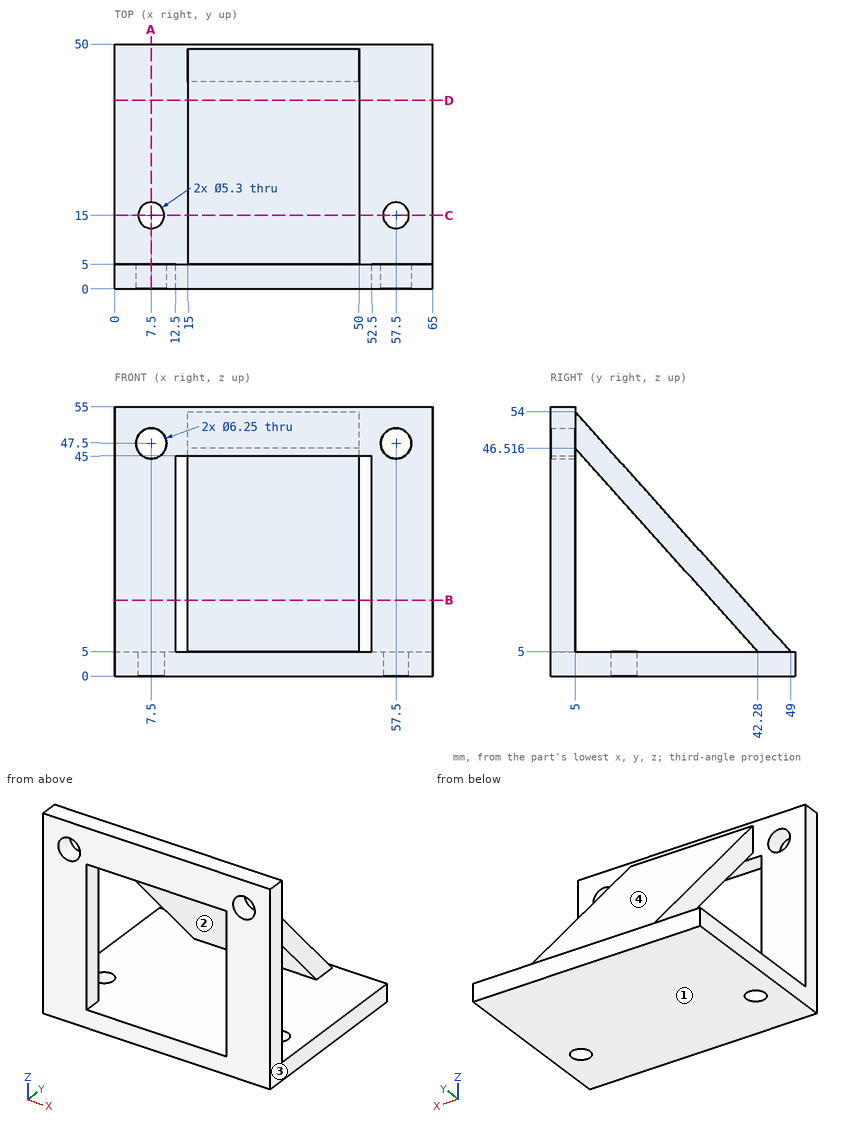
Answer from the drawing. Dimensions are ordinates in mm from the lowest x, y and z of the part. Give positions to 0.01 mm unless a question says otherwise; leave off trailing zeros. Write each loop counter-clockwise with the first axis right and the second up, starting at its lowest first coordinate (ties: lowest second). Pieces come first, ordered by that corner, then holes. Notation, with made-up numbers: (67.5, 52.5) - (110.5, 52.5) arc R22 cw to (110.5, 83.5) - close; hole circle Ø7 at (28, 28.25). An arc over 180 degrees is marked (long way). One line per item, written item: value. Start each with the question number.
1. Given pin 1 (12 mm diameter, centred on x = 40.5, y = 41.5, fed in from +Z) (1 decimal); pin 2 (1 mm diameter, centred on x = 55, z = 33, fed in from +Y); pin 3 (6 mm diameter, centred on x = 31.5, y = 26.5, fed in from +Z), each flat-ended and moving along its own axis, determine where each tip first touches the part or whether it passes through.
2. Find section B-B (z = 15.5). Write down the section's boundary in (x, y), then the cut area to 3 significant figures.
3. Find section A-A (x = 7.5). State how many separate pieces and enclosed holes the cut face has, then the cut area to 3 significant figures.
4. Find section C-C (y = 15). Write down the section's boundary in (x, z).
5. Consider probe 1 along X at (y, z) = (3.15, 47.5) (1 decimal); probe 2 along X at (y, z) = (3, 19.5); probe 3 along Z at (x, y) = (57.5, 2.55) (1 decimal). Determine where each line is inside the solid, lowest interval first.
6. Find section D-D (y = 38.5). Write down the section's boundary in (x, z).
7. For a pull along Z with two mould halves and no side action, classify the marked faces 1, 2, 3 and 4 as +Z half, -Z half, draft (parallel to the pull), parting line (faces both ways), or undercut.
Geometry results:
1. pin 1: z = 20
1. pin 2: y = 5
1. pin 3: z = 33.4
2. outline: (0, 0) - (12.5, 0) - (12.5, 5) - (0, 5) - close; (15, 32.85) - (50, 32.85) - (50, 39.57) - (15, 39.57) - close; (52.5, 0) - (65, 0) - (65, 5) - (52.5, 5) - close
2. area: 360 mm2
3. separate pieces: 3
3. enclosed holes: 0
3. area: 442 mm2
4. outline: (0, 0) - (4.85, 0) - (4.85, 5) - (0, 5) - close; (10.15, 0) - (54.85, 0) - (54.85, 5) - (10.15, 5) - close; (15, 35.38) - (50, 35.38) - (50, 42.86) - (15, 42.86) - close; (60.15, 0) - (65, 0) - (65, 5) - (60.15, 5) - close
5. probe 1: 0 to 4.4, 10.6 to 54.4, 60.6 to 65
5. probe 2: 0 to 12.5, 52.5 to 65
5. probe 3: 0 to 44.4, 50.6 to 55
6. outline: (0, 0) - (65, 0) - (65, 5) - (0, 5) - close; (15, 9.21) - (50, 9.21) - (50, 16.69) - (15, 16.69) - close
7. face 1: -Z half
7. face 2: undercut
7. face 3: draft
7. face 4: +Z half
